Read the model definition and answer for the solid it produces. Units are mm, in the model's axes. Give positions to 0.01 mm unless a question says otherwise; leave off trailing zeros. Loops run counter-clockwise (first coordinate to the right, second up) from the corner with the lowest first, then second, coordinate; pieces in that order, holes last. Notation, with made-up numbers: (85.5, -0.75) -> (141.5, -0.75) arc R26 ccw to (141.5, 36.25) -> close; hole circle Ø9 at (68.25, 37.25). An arc over 180 degrees is marked (long way). Answer as CSV lines item,"result". Start each with the question number.
Autodesk Inventor part; units mm, degrees
ref_plane "YZ Plane" through (0, 0, 0) normal (1, 0, 0) x (0, 1, 0)
ref_plane "XZ Plane" through (0, 0, 0) normal (0, 1, 0) x (-1, 0, 0)
ref_plane "XY Plane" through (0, 0, 0) normal (0, 0, 1) x (1, 0, 0)
sketch "スケッチ1" plane through (0, 0, 0) normal (1, 0, 0) x (0, 1, 0)
  line L0 (-64.254, -635.7138) -> (-64.254, 672.2862)
  line L1 (-64.254, -533.7138) -> (340.746, -533.7138)
  line L2 (340.746, -533.7138) -> (340.746, -513.7138)
  line L3 (340.746, -513.7138) -> (-64.254, -513.7138)
  line L4 (-64.254, -513.7138) -> (-64.254, -533.7138)
  circle A0 centre (-29.074, -486.7138) radius 21
  circle A1 centre (-29.074, -444.7138) radius 16
  circle A2 centre (-29.074, -444.7138) radius 13.68
  line L5 (-84.254, -635.7138) -> (-64.254, -635.7138)
  line L6 (-84.254, -635.7138) -> (-64.254, -635.7138)
  line L7 (-84.254, -635.7138) -> (399.746, -635.7138)
  line L8 (399.746, -635.7138) -> (399.746, -655.7138)
  line L9 (399.746, -655.7138) -> (-84.254, -655.7138)
  line L10 (-84.254, -655.7138) -> (-84.254, -635.7138)
  line L11 (-9.074, 672.2862) -> (10.1017, 677.9687)
  line L12 (10.1017, 677.9687) -> (395.949, -624.0627)
  line L13 (395.949, -624.0627) -> (376.7733, -629.7453)
  line L14 (376.7733, -629.7453) -> (-9.074, 672.2862)
  line L15 (-84.254, 672.2862) -> (-84.254, -635.7138)
  line L16 (-84.254, -428.7138) -> (-29.074, -428.7138)
  line L17 (-8.074, -486.7138) -> (-8.074, -533.7138)
  line L18 (-8.074, -486.7138) -> (-8.074, -428.7138)
  line L19 (-8.074, -428.7138) -> (-29.074, -428.7138)
  circle A3 centre (-74.254, -440.7138) radius 1.5
  circle A4 centre (-74.254, -450.7138) radius 1.5
  line L20 (-29.074, -460.7138) -> (-84.254, -460.7138)
  circle A5 centre (-54.254, -523.7138) radius 1.5
  circle A6 centre (-34.254, -523.7138) radius 1.5
  line L21 (-64.254, -533.7138) -> (-84.254, -533.7138)
  circle A7 centre (-74.254, -523.7138) radius 1.5
  circle A8 centre (-74.254, -503.7138) radius 1.5
  circle A9 centre (-29.074, 656.2862) radius 16
  line L22 (-64.254, 672.2862) -> (-84.254, 672.2862)
  line L23 (-84.254, 672.2862) -> (-29.074, 672.2862)
  line L24 (-29.074, 640.2862) -> (-84.254, 640.2862)
  line L25 (-29.074, 672.2862) -> (-9.074, 672.2862)
  circle A10 centre (-29.074, 656.2862) radius 7.5
  line L26 (-29.074, 640.2862) -> (0.4089, 640.2862)
  circle A11 centre (-74.254, 660.2862) radius 1.5
  circle A12 centre (-74.254, 650.2862) radius 1.5
  circle A13 centre (3.3551, 665.5396) radius 1.5
  circle A14 centre (6.1964, 655.9517) radius 1.5
  line L27 (0.4089, 640.2862) -> (19.5847, 645.9687)
  line L28 (-64.254, -595.7138) -> (-44.254, -635.7138)
  line L29 (-44.254, -635.7138) -> (-44.254, -655.7138)
  line L30 (-64.254, -595.7138) -> (-84.254, -595.7138)
  circle A15 centre (-74.254, -625.7138) radius 1.5
  circle A16 centre (-74.254, -615.7138) radius 1.5
  circle A17 centre (-74.254, -605.7138) radius 1.5
  circle A18 centre (-74.254, -645.7138) radius 1.5
  circle A19 centre (-64.254, -645.7138) radius 1.5
  circle A20 centre (-54.254, -645.7138) radius 1.5
  line L31 (-84.254, -635.7138) -> (-84.254, -595.7138)
  line L32 (369.746, -635.7138) -> (369.746, -655.7138)
  line L33 (368.2494, -600.9817) -> (387.4252, -595.2991)
  line L34 (376.7733, -629.7453) -> (378.5421, -635.7138)
  line L35 (395.949, -624.0627) -> (399.746, -635.7138)
  circle A21 centre (379.746, -645.7138) radius 1.5
  circle A22 centre (389.746, -645.7138) radius 1.5
  circle A23 centre (383.5199, -617.3161) radius 1.5
  circle A24 centre (380.6786, -607.7283) radius 1.5
  circle A25 centre (320.746, -523.7138) radius 1.5
  circle A26 centre (330.746, -523.7138) radius 1.5
  line L36 (340.746, -513.7138) -> (342.3883, -513.7138)
  line L37 (340.746, -533.7138) -> (348.3151, -533.7138)
  line L38 (342.3883, -513.7138) -> (363.248, -513.7138)
  circle A27 centre (355.6752, -523.3551) radius 1.5
  circle A28 centre (358.5165, -532.9429) radius 1.5
  line L39 (351.7699, -545.3721) -> (370.9457, -539.6895)
  line L40 (310.746, -513.7138) -> (310.746, -533.7138)
  line L41 (368.2494, -600.9817) -> (369.746, -635.7138)
  point P0 (0, 0)
  point P1 (-387.254, -203.3804)
  point P2 (-64.254, -513.7138)
  point P3 (386.3612, -626.904)
  dimension "d1" = 42
  dimension "d0" = 20
  dimension "d2" = 32
  dimension "d3" = 27.36
  dimension "d4" = 35.18
  dimension "d5" = 35.18
  dimension "d6" = 27
  dimension "d7" = 42
  dimension "d8" = 191
  dimension "d9" = 20
  dimension "d10" = 484
  dimension "d11" = 3
  dimension "d12" = 3
  dimension "d13" = 10
  dimension "d14" = 10
  dimension "d15" = 10
  dimension "d16" = 10
  dimension "d17" = 3
  dimension "d18" = 3
  dimension "d19" = 10
  dimension "d20" = 20
  dimension "d21" = 10
  dimension "d22" = 10
  dimension "d23" = 3
  dimension "d24" = 3
  dimension "d25" = 10
  dimension "d26" = 20
  dimension "d27" = 10
  dimension "d28" = 10
  dimension "d29" = 20
  dimension "d30" = 32
  dimension "d31" = 35.18
  dimension "d32" = 20
  dimension "d33" = 1358
  dimension "d34" = 91.543
  dimension "d35" = 405
  dimension "d36" = 15
  dimension "d37" = 3
  dimension "d38" = 3
  dimension "d39" = 10
  dimension "d40" = 10
  dimension "d41" = 10
  dimension "d42" = 10
  dimension "d43" = 3
  dimension "d44" = 3
  dimension "d45" = 10
  dimension "d46" = 10
  dimension "d47" = 10
  dimension "d48" = 10
  dimension "d49" = 40
  dimension "d50" = 3
  dimension "d51" = 3
  dimension "d52" = 3
  dimension "d53" = 3
  dimension "d54" = 3
  dimension "d55" = 3
  dimension "d56" = 10
  dimension "d57" = 10
  dimension "d58" = 10
  dimension "d59" = 10
  dimension "d60" = 10
  dimension "d61" = 10
  dimension "d62" = 10
  dimension "d63" = 10
  dimension "d64" = 10
extrude "押し出し1" add sketch "スケッチ1" against normal blind 2 contours L7 L8 L9 L32 | L34 L13 L35 L7 | L33 L12 L13 L14
fillet "フィレット1" radius 2 7 edges at (-1, 368.2494, -600.9817) (-1, 378.5421, -635.7138) (-1, 369.746, -635.7138) (-1, 369.746, -655.7138) (-1, 399.746, -655.7138) (-1, 399.746, -635.7138) (-1, 387.4252, -595.2991)
equation "\"d14\" = d15"
equation "\"d21\" = d19"
equation "\"d22\" = d19"
equation "\"d27\" = d25"
equation "\"d28\" = d25"
equation "\"d31\" = d4"
equation "\"d41\" = d39"
equation "\"d42\" = d39"
equation "\"d46\" = d45"
equation "\"d47\" = d45"
equation "\"d48\" = d45"
equation "\"d57\" = d56"
equation "\"d58\" = d56"
equation "\"d59\" = d56"
equation "\"d60\" = d56"
equation "\"d61\" = d56"
equation "\"d62\" = d56"
equation "\"d63\" = d56"
equation "\"d64\" = d62"
properties part number "dribl-v1-Plate-10" material "アルミニウム 6061"
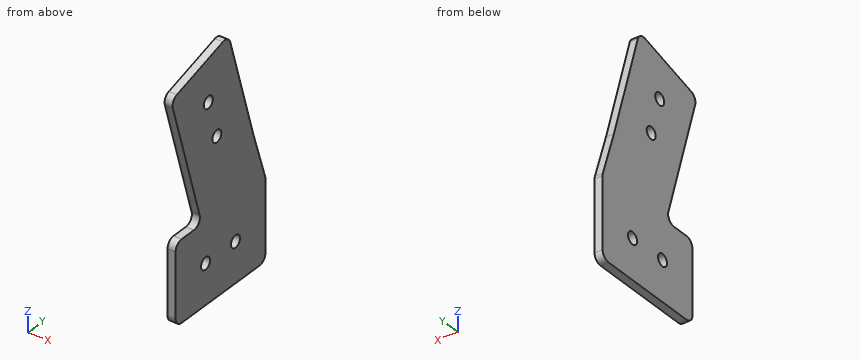
(1) Find section A-A on z = -608.5. Write down the section's boundary in (x, y).
(2) Find section C-C on x = -0.3. Write down the section's boundary in (y, z).
(3) Find section B-B on y = 374.5. Write down the section's boundary in (x, z), then the cut area to 3 significant figures.
(4) Find the intervals of material crossed by line 1 along Z through (x, y) = (-1.35, 379.5); line 2 along Z through (x, y) = (-0.8, 384.5); line 3 along Z through (x, y) = (-0.5, 384) (3 decimals), in increasing order. Write a range as from..to.
(5) Find section D-D on z = -642.5. Write down the section's boundary in (x, y), then the cut area to 3 significant figures.
(6) This flat-tipped pin is pushed along its axis until it touches: P1, Ø1, axis at x = -1.5, z = -643, coming from the -Y side. Where does it stop, or does it pass through?
Answer block:
1,outline,"(-2, 370.48) -> (0, 370.48) -> (0, 379.39) -> (-2, 379.39) -> close; (-2, 381.96) -> (0, 381.96) -> (0, 391.34) -> (-2, 391.34) -> close"
2,outline,"(368.82, -602.9) -> (376.77, -629.75) -> (377.78, -633.15) arc R2 cw to (375.86, -635.71) -> (371.75, -635.71) arc R2 ccw to (369.75, -637.71) -> (369.75, -653.71) arc R2 ccw to (371.75, -655.71) -> (397.75, -655.71) arc R2 ccw to (399.75, -653.71) -> (399.75, -636.03) arc R2 ccw to (399.65, -635.41) -> (395.95, -624.06) -> (387.99, -597.22) arc R2 ccw to (385.51, -595.87) -> (370.17, -600.41) arc R2 ccw to start; hole circle Ø3 at (379.75, -645.71); hole circle Ø3 at (380.68, -607.73); hole circle Ø3 at (383.52, -617.32); hole circle Ø3 at (389.75, -645.71)"
3,outline,"(-2, -655.71) -> (0, -655.71) -> (0, -635.71) -> (-2, -635.71) -> close; (-2, -622.07) -> (0, -622.07) -> (0, -599.13) -> (-2, -599.13) -> close"
3,area,"85.9 mm2"
4,line 1,"z = -655.71..-647.19, -644.23..-608.66, -606.8..-597.65"
4,line 2,"z = -655.71..-618.45, -616.18..-596.17"
4,line 3,"z = -655.714..-618.737, -615.895..-596.314"
5,outline,"(-2, 369.75) -> (0, 369.75) -> (0, 399.75) -> (-2, 399.75) -> close"
5,area,"60.0 mm2"
6,P1,"stops at y = 369.75"
